Check sheet for the modelled part. Datum: model origin and axes. Units: mm. A direction names the side the tool comes from. Round coordinates to 2 decimals unless told otherwise and drop trailing zeros. Write each loop counter-clockwise with the first axis right and the second up, starting at its lowest first coordinate (ties: lowest second). Pieces come first, ordered by that corner, then holes. Notation, with made-up numbers: M -33.75,66 L -22.75,66 A28 ccw -22.75,86 Z; hole C 75.5,-18.75 d8. An arc over 180 degrees is marked long. Put each result on its own line as item: value.
```python
from build123d import *

# Parameters (mm, degrees)
SKETCH1_W           = 18
SKETCH1_H           = 18
BOSS_EXTRUDE1_DEPTH = 30
FILLET1_R           = 2
SKETCH2_R           = 5
CUT_EXTRUDE1_DEPTH  = 12
SKETCH3_R           = 5.5
BOSS_EXTRUDE2_DEPTH = 10
SKETCH4_R           = 4
BOSS_EXTRUDE3_DEPTH = 5
SKETCH5_R           = 3
CUT_EXTRUDE2_DEPTH  = 3
SKETCH6_R           = 1.5
CUT_EXTRUDE3_DEPTH  = 19
CHAMFER1_SIZE       = 2
FILLET2_R           = 1
SKETCH7_R           = 1.5
CUT_EXTRUDE4_DEPTH  = 32.320919527
CHAMFER2_SIZE       = 0.3


with BuildPart() as part:
    # Sketch1 → Boss-Extrude1 (new body)
    with BuildSketch(Plane.XY):
        Rectangle(SKETCH1_W, SKETCH1_H)
    extrude(amount=BOSS_EXTRUDE1_DEPTH)

    # Fillet1
    fillet1_edges = [part.edges().sort_by_distance(p)[0] for p in [
        (-9, 9, 15),
        (9, 9, 15),
        (9, -9, 15),
        (-9, -9, 15),
    ]]
    fillet(fillet1_edges, radius=FILLET1_R)

    # Sketch2 → Cut-Extrude1 (cut)
    with BuildSketch(Plane(origin=(0, 0, 0), x_dir=(-1, 0, 0), z_dir=(0, 0, -1))):
        Circle(SKETCH2_R)
    cut_extrude1 = extrude(amount=-CUT_EXTRUDE1_DEPTH, mode=Mode.SUBTRACT)

    # Mirror1: Cut-Extrude1 across plane
    add(cut_extrude1.mirror(Plane.XY.offset(15)), mode=Mode.SUBTRACT)

    # Sketch3 → Boss-Extrude2 (add)
    with BuildSketch(Plane(origin=(0, 9, 0), x_dir=(1, 0, 0), z_dir=(0, 1, 0))):
        with Locations((0, -15)):
            Circle(SKETCH3_R)
    extrude(amount=BOSS_EXTRUDE2_DEPTH)

    # Sketch4 → Boss-Extrude3 (add)
    with BuildSketch(Plane(origin=(0, 19, 0), x_dir=(1, 0, 0), z_dir=(0, 1, 0))):
        with Locations(Location((0, -15, 0), (0, 0, 180))):
            Circle(SKETCH4_R)
    extrude(amount=BOSS_EXTRUDE3_DEPTH)

    # Sketch5 → Cut-Extrude2 (cut)
    with BuildSketch(Plane(origin=(0, 24, 0), x_dir=(1, 0, 0), z_dir=(0, 1, 0))):
        with Locations(Location((0, -15, 0), (0, 0, 180))):
            Circle(SKETCH5_R)
    extrude(amount=-CUT_EXTRUDE2_DEPTH, mode=Mode.SUBTRACT)

    # Sketch6 → Cut-Extrude3 (cut)
    with BuildSketch(Plane(origin=(0, 21, 0), x_dir=(1, 0, 0), z_dir=(0, 1, 0))):
        with Locations(Location((0, -15, 0), (0, 0, 180))):
            Circle(SKETCH6_R)
    extrude(amount=-CUT_EXTRUDE3_DEPTH, mode=Mode.SUBTRACT)

    # Chamfer1
    # the kernel refuses this chamfer: 2 mm, written as the material it takes off along each edge
    with BuildSketch(Plane(origin=(0, 21, 15), x_dir=(-1, 0, 0), z_dir=(0, 0, -1))) as chamfer1_piece_1_section:
        Polygon((1.5 + CHAMFER1_SIZE, 0), (1.5, -CHAMFER1_SIZE), (1.5, 0), align=None)
    chamfer1_piece_1 = revolve(axis=Axis((0, 21, 15), (0, 1, 0)), mode=Mode.PRIVATE)
    chamfer1_piece_1 = chamfer1_piece_1 & Plane(origin=(0, 19.742805432, 15), x_dir=(-1, 0, 0), z_dir=(0, 1, 0)) * Cylinder(3, 14, mode=Mode.PRIVATE)
    add(chamfer1_piece_1, mode=Mode.SUBTRACT)

    # Fillet2
    fillet2_edges = [part.edges().sort_by_distance(p)[0] for p in [
        (-5.5, 9, 15),
    ]]
    fillet(fillet2_edges, radius=FILLET2_R)

    # Sketch7 → Cut-Extrude4 (cut, through all)
    with BuildSketch(Plane(origin=(0, 0, 12), x_dir=(-1, 0, 0), z_dir=(0, 0, -1))):
        Circle(SKETCH7_R)
    extrude(amount=-CUT_EXTRUDE4_DEPTH, mode=Mode.SUBTRACT)

    # Chamfer2
    chamfer2_edges = [part.edges().sort_by_distance(p)[0] for p in [
        (9, 0, 0),
        (9, 0, 30),
        (-9, 0, 0),
        (0, 9, 0),
        (0, -9, 0),
        (-8.414213562, 8.414213562, 0),
        (8.414213562, 8.414213562, 0),
        (-8.414213562, -8.414213562, 0),
        (8.414213562, -8.414213562, 0),
        (0, -9, 30),
        (-9, 0, 30),
        (0, 9, 30),
        (-8.414213562, 8.414213562, 30),
        (8.414213562, 8.414213562, 30),
        (-8.414213562, -8.414213562, 30),
        (8.414213562, -8.414213562, 30),
        (-5.5, 19, 15),
        (4, 24, 15),
    ]]
    chamfer(chamfer2_edges, length=CHAMFER2_SIZE)


solid = part.part
```
1. Cross-section at B-B (z = 25.25). Enter the section's corners in (x, y), then the cut area to 3 significant figures.
Computed values:
outline: M -9,-7 A2 ccw -7,-9 L 7,-9 A2 ccw 9,-7 L 9,7 A2 ccw 7,9 L -7,9 A2 ccw -9,7 Z; hole C 0,0 d10
area: 242 mm2
2. Depth check by flat-ended pin: pin 1 Ø8 at (x, y) = (0.5, -1.5) entering from +Z; pin 2 Ø1.5 at (x, z) = (-5, 23) entering from +Y; pin 3 Ø4 at (x, y) = (5.5, 15.5) entering from +Z; pin 4 Ø0.9 at (x, z) = (0.5, 15.5) entering from +Y. Enter the tip coordinate at first touch or a pass-through.
Computed values:
pin 1: stops at z = 30
pin 2: stops at y = 9
pin 3: stops at z = 19.24
pin 4: stops at y = 2
3. Cross-section at D-D (y = 13). Enter the section's corners in (x, z).
Computed values:
outline: C 0,15 d11; hole C 0,15 d3
4. Scan lines: probe 1 along Y at (x, z) = (0, 14.25); probe 2 along Z at (x, y) = (0, 22.8); probe 3 along Y at (x, z) = (0, 5.5). Record each from-to range of solid material in increasing order.
Computed values:
probe 1: y = -9 to -1.5, 1.5 to 2
probe 2: z = 11 to 12, 18 to 19
probe 3: y = -9 to -5, 5 to 9
5. Release check for a two-part mould opening along Y. For faces 1 (the cylindrical face through (1.08, -4.88, 24.08)), 2 (the cylindrical face through (8.43, 8.4, 15.21)), 3 (the flat face through (1.2, 1.2, 12)), 4 (the cylindrical face through (8.4, -8.43, 15.21)) record: +Y half, -Y half, draft (parallel to the pull), parting line (faces both ways), or undercut.
Computed values:
face 1: undercut
face 2: +Y half
face 3: undercut
face 4: -Y half
6. Access from +Z, -Z, +X, -X, +Y, -Y to the whole of each face (thin tool, end or side, straight path). Record for faces 5 (the cylindrical face through (1.5, 0.07, 14.96)), 6 (the cylindrical face through (1.11, 10.62, 16.01)).
Computed values:
face 5: +Z, -Z
face 6: +Y
7. Cross-section at A-A (y = 0). Enter the section's corners in (x, z).
Computed values:
outline: M -9,0.3 L -8.7,0 L -5,0 L -5,12 L -1.5,12 L -1.5,18 L -5,18 L -5,30 L -8.7,30 L -9,29.7 Z; M 1.5,12 L 5,12 L 5,0 L 8.7,0 L 9,0.3 L 9,29.7 L 8.7,30 L 5,30 L 5,18 L 1.5,18 Z
